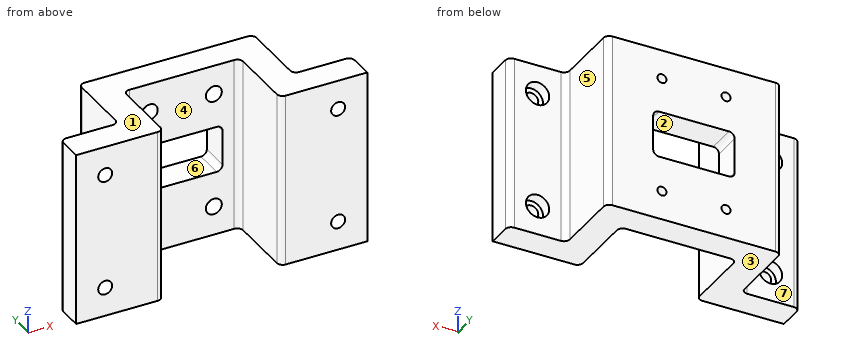
```python
from build123d import *

# Parameters (mm, degrees)
SKETCH2_W                        = 60
SKETCH2_H                        = 60
BOSS_EXTRUDE1_DEPTH              = 10
SKETCH7_W                        = 28
SKETCH7_H                        = 16
CUT_EXTRUDE2_DEPTH               = 44.588989435
FILLET2_R                        = 2
CBORE_FOR_M2_5_SHCS2_D           = 3.1
CBORE_FOR_M2_5_SHCS2_CBORE_D     = 5.5
CBORE_FOR_M2_5_SHCS2_CBORE_DEPTH = 2.5
MOVE_FACE1_BY                    = 3.5
MOVE_FACE1_2_BY                  = 3.5
MOVE_FACE1_3_BY                  = 3.5
MOVE_FACE1_4_BY                  = 3.5
SKETCH11_W                       = 10
SKETCH11_H                       = 25.4
BOSS_EXTRUDE2_DEPTH              = 60
SKETCH12_W                       = 20
SKETCH12_H                       = 60
BOSS_EXTRUDE3_DEPTH              = 10
CBORE_FOR_M4_SHCS1_D             = 4.8
CBORE_FOR_M4_SHCS1_CBORE_D       = 8
CBORE_FOR_M4_SHCS1_CBORE_DEPTH   = 4
FILLET5_R                        = 2


with BuildPart() as part:
    # Sketch2 → Boss-Extrude1 (new body)
    with BuildSketch(Plane(origin=(0, 0, 0), x_dir=(1, 0, 0), z_dir=(0, 1, 0))):
        Rectangle(SKETCH2_W, SKETCH2_H)
    extrude(amount=BOSS_EXTRUDE1_DEPTH)

    # Sketch7 → Cut-Extrude2 (cut, through all)
    with BuildSketch(Plane(origin=(0, 10, 0), x_dir=(1, 0, 0), z_dir=(0, 1, 0))):
        Rectangle(SKETCH7_W, SKETCH7_H)
    extrude(amount=-CUT_EXTRUDE2_DEPTH, mode=Mode.SUBTRACT)

    # Fillet2
    fillet2_edges = [part.edges().sort_by_distance(p)[0] for p in [
        (-14, 5, 8),
        (-14, 5, -8),
        (14, 5, -8),
        (14, 5, 8),
    ]]
    fillet(fillet2_edges, radius=FILLET2_R)

    # CBORE for M2.5 SHCS2 (through all)
    with Locations(Plane(origin=(0, 0, 0), x_dir=(-1, 0, 0), z_dir=(0, -1, 0))):
        with Locations((11, -20), (-11, -20), (11, 20), (-11, 20)):
            CounterBoreHole(CBORE_FOR_M2_5_SHCS2_D / 2, CBORE_FOR_M2_5_SHCS2_CBORE_D / 2, CBORE_FOR_M2_5_SHCS2_CBORE_DEPTH)

    # Move Face1: a face moved inward by 3.5
    extrude(part.faces().sort_by_distance((11, 2.5, -17.8))[0], amount=MOVE_FACE1_BY, dir=(0, 1, 0), mode=Mode.SUBTRACT)

    # Move Face1 2: a face moved inward by 3.5
    extrude(part.faces().sort_by_distance((-11, 2.5, -17.8))[0], amount=MOVE_FACE1_2_BY, dir=(0, 1, 0), mode=Mode.SUBTRACT)

    # Move Face1 3: a face moved inward by 3.5
    extrude(part.faces().sort_by_distance((11, 2.5, 22.2))[0], amount=MOVE_FACE1_3_BY, dir=(0, 1, 0), mode=Mode.SUBTRACT)

    # Move Face1 4: a face moved inward by 3.5
    extrude(part.faces().sort_by_distance((-11, 2.5, 22.2))[0], amount=MOVE_FACE1_4_BY, dir=(0, 1, 0), mode=Mode.SUBTRACT)

    # Sketch11 → Boss-Extrude2 (add)
    with BuildSketch(Plane(origin=(0, 0, -30), x_dir=(-1, 0, 0), z_dir=(0, 0, -1))):
        with Locations((-25, -12.7)):
            Rectangle(SKETCH11_W, SKETCH11_H)
    boss_extrude2 = extrude(amount=-BOSS_EXTRUDE2_DEPTH)

    # Sketch12 → Boss-Extrude3 (add)
    with BuildSketch(Plane.XZ.offset(25.4)):
        with Locations((40, 0)):
            Rectangle(SKETCH12_W, SKETCH12_H)
    boss_extrude3 = extrude(amount=-BOSS_EXTRUDE3_DEPTH)

    # CBORE for M4 SHCS1 (through all)
    with Locations(Plane(origin=(0, -15.4, 0), x_dir=(1, 0, 0), z_dir=(0, 1, 0))):
        with Locations((40, 20), (40, -20)):
            cbore_for_m4_shcs1 = CounterBoreHole(CBORE_FOR_M4_SHCS1_D / 2, CBORE_FOR_M4_SHCS1_CBORE_D / 2, CBORE_FOR_M4_SHCS1_CBORE_DEPTH)

    # Mirror1: Boss-Extrude2, Boss-Extrude3, CBORE for M4 SHCS1 across plane
    add(boss_extrude2.mirror(Plane(origin=(0, 0, 0), x_dir=(0, 0, 1), z_dir=(1, 0, 0))))
    add(boss_extrude3.mirror(Plane(origin=(0, 0, 0), x_dir=(0, 0, 1), z_dir=(1, 0, 0))))
    add(cbore_for_m4_shcs1.mirror(Plane(origin=(0, 0, 0), x_dir=(0, 0, 1), z_dir=(1, 0, 0))), mode=Mode.SUBTRACT)

    # Fillet5
    fillet5_edges = [part.edges().sort_by_distance(p)[0] for p in [
        (50, -15.4, 0),
        (30, -15.4, 0),
        (30, 10, 0),
        (-20, 0, 0),
        (-20, -25.4, 0),
        (-30, -15.4, 0),
        (-50, -15.4, 0),
        (-30, 10, 0),
        (20, 0, 0),
        (20, -25.4, 0),
    ]]
    fillet(fillet5_edges, radius=FILLET5_R)


solid = part.part
```
CAD build for the part. Positions are in the model's coordinates, mm. Face numbers are marked on the shaded views. A direction names the side the tool comes from. Round coordinates to 2 decimals unless told otherwise and drop trailing zeros. Write each loop counter-clockwise with the first axis right and the second up, starting at its lowest first coordinate (ties: lowest second). Pieces come first, ordered by that corner, then holes. Notation, with made-up numbers: (31, -0.75) -> (56, -0.75) arc R35 ccw to (56, 33.25) -> close; hole circle Ø2 at (0.25, -3.75). An arc over 180 degrees is marked (long way). Answer in a Markdown table with one row per item. Add a question column.
Item 1: Mould opens along Z. For the marked faces 1, 2, 3 and 4 say: pulls with the +Z half, pulls with the -Z half, needs draft (parallel to the pull), parting line crosses it, or undercut.
Item 2: Drill centre lines: line 1 (X direction, y = -22.7, z = -20); line 2 (X direction, y = -17.75, z = 20); line 3 (Z direction, x = -40, y = -22.9). Where is each one in solid material? Low to high. Write a range as from..to.
Item 3: Saw through at C-C, the plane x = -40. Write the cut outline in (y, z), then the cut area to 3 significant figures.
Item 4: Saw through at D-D, the plane z = 25. Write the cut outline in (x, y).
Item 5: Saw through at A-A, the plane y = -21. Write the cut outline in (x, z), then the cut area to 3 significant figures.
Item 6: Drop flat-ended pins along their axis: pin 1 Ø1 at (x, z) = (37.5, -18) entering from +Y; pin 2 Ø10 at (x, z) = (-1.5, -13) entering from -Y; pin 3 Ø9 at (x, z) = (40, 20) entering from +Y. Give the stop position or say it passes through.
Item 7: Saw through at B-B, the plane x = -11. Write the cut outline in (y, z), then the cut area to 3 significant figures.
Item 8: Which spindle directions (+Z, -Z, +X, -X, +Y, -Y) get a long thin tool onto all of the face, cutting with end or side? Do the marked faces 5, 6 and 7. Say none if no direction does.
Findings below:
| question | item | result |
|---|---|---|
| 1 | face 1 | pulls with the +Z half |
| 1 | face 2 | undercut |
| 1 | face 3 | pulls with the -Z half |
| 1 | face 4 | needs draft |
| 2 | line 1 | x = -50..-42.4, -37.6..-20, 20..37.6, 42.4..50 |
| 2 | line 2 | x = -50..-44, -36..-20, 20..36, 44..50 |
| 2 | line 3 | z = -30..-22.4, -17.6..17.6, 22.4..30 |
| 3 | outline | (-25.4, -30) -> (-15.4, -30) -> (-15.4, -24) -> (-19.4, -24) -> (-19.4, -22.4) -> (-25.4, -22.4) -> close; (-25.4, -17.6) -> (-19.4, -17.6) -> (-19.4, -16) -> (-15.4, -16) -> (-15.4, 16) -> (-19.4, 16) -> (-19.4, 17.6) -> (-25.4, 17.6) -> close; (-25.4, 22.4) -> (-19.4, 22.4) -> (-19.4, 24) -> (-15.4, 24) -> (-15.4, 30) -> (-25.4, 30) -> close |
| 3 | area | 478 mm^2 |
| 4 | outline | (-50, -25.4) -> (-22, -25.4) arc R2 ccw to (-20, -23.4) -> (-20, -2) arc R2 cw to (-18, 0) -> (18, 0) arc R2 cw to (20, -2) -> (20, -23.4) arc R2 ccw to (22, -25.4) -> (50, -25.4) -> (50, -17.4) arc R2 ccw to (48, -15.4) -> (32, -15.4) arc R2 cw to (30, -13.4) -> (30, 8) arc R2 ccw to (28, 10) -> (-28, 10) arc R2 ccw to (-30, 8) -> (-30, -13.4) arc R2 cw to (-32, -15.4) -> (-48, -15.4) arc R2 ccw to (-50, -17.4) -> close |
| 5 | outline | (-50, -30) -> (-20, -30) -> (-20, 30) -> (-50, 30) -> close; (20, -30) -> (50, -30) -> (50, 30) -> (20, 30) -> close; hole circle Ø4.8 at (-40, -20); hole circle Ø4.8 at (-40, 20); hole circle Ø4.8 at (40, -20); hole circle Ø4.8 at (40, 20) |
| 5 | area | 3,530 mm^2 |
| 6 | pin 1 | stops at y = -19.4 |
| 6 | pin 2 | stops at y = 0 |
| 6 | pin 3 | stops at y = -15.4 |
| 7 | outline | (0, -30) -> (10, -30) -> (10, -21.55) -> (6, -21.55) -> (6, -22.75) -> (0, -22.75) -> close; (0, -17.25) -> (6, -17.25) -> (6, -18.45) -> (10, -18.45) -> (10, -8) -> (0, -8) -> close; (0, 8) -> (10, 8) -> (10, 18.45) -> (6, 18.45) -> (6, 17.25) -> (0, 17.25) -> close; (0, 22.75) -> (6, 22.75) -> (6, 21.55) -> (10, 21.55) -> (10, 30) -> (0, 30) -> close |
| 7 | area | 349 mm^2 |
| 8 | face 5 | +Z, -Z, +X, +Y |
| 8 | face 6 | +Y, -Y |
| 8 | face 7 | +Z, -Z, -X, +Y |
